from build123d import *

# Parameters (mm, degrees)
SKETCH1_W                  = 35.3
SKETCH1_H                  = 24
BOSS_EXTRUDE1_DEPTH        = 1
F_3_5_3_5_DIAMETER_HOLE1_D = 3.5
SKETCH5_W                  = 7.129651431
SKETCH5_H                  = 6
BOSS_EXTRUDE2_DEPTH        = 0.7


with BuildPart() as part:
    # Sketch1 → Boss-Extrude1 (new body)
    with BuildSketch(Plane(origin=(0, 0, 0), x_dir=(1, 0, 0), z_dir=(0, 1, 0))):
        Rectangle(SKETCH1_W, SKETCH1_H)
    extrude(amount=BOSS_EXTRUDE1_DEPTH)

    # Ø3.5 (3.5) Diameter Hole1 (through all)
    with Locations(Plane(origin=(0, 1, 0), x_dir=(1, 0, 0), z_dir=(0, 1, 0))):
        with Locations((-3.75, 8.7), (14.35, -8.7)):
            Hole(F_3_5_3_5_DIAMETER_HOLE1_D / 2)

    # Sketch5 → Boss-Extrude2 (add)
    with BuildSketch(Plane.XZ):
        with Locations((18.431222248, -1)):
            Rectangle(SKETCH5_W, SKETCH5_H)
    extrude(amount=BOSS_EXTRUDE2_DEPTH)


solid = part.part
For this review, take the finished solid that the model builds, in its own axes (mm). A direction names the side the tool comes from. Give positions to 0.01 mm unless a question says otherwise; leave off trailing zeros. Loops run counter-clockwise (first coordinate to the right, second up) from the corner with the lowest first, then second, coordinate; pieces in that order, holes last. Notation, with made-up numbers: M -38,-28.5 L 7,-28.5 A18 cw 7,-6.5 Z; hole C 75,-11 d3. An arc over 180 degrees is marked long. Put each result on its own line as item: value. Start each with the question number.
(1) Add section C-C, the plane x = 14.35. Write out the cut boundary in (y, z), then the cut area to 3 significant figures.
(2) Add section A-A, the plane z = -8.7. Write out the cut boundary in (x, y).
(3) Add section B-B, the plane y = 0.5. Write out the cut boundary in (x, z), then the cut area to 3 significant figures.
(4) The part is to be moulded in two halves that separate along X. For faces 3 (the cylindrical face through (-2, 0.49, -8.78)), 4 (the flat face through (-17.65, 0.5, 0.2)), 5 (the flat face through (0, 0, 0)), 6 (the cylindrical face through (15.64, 0.49, 7.52)), say which applies: +X half, -X half, draft (parallel to the pull), parting line (faces both ways), or undercut.
(5) Wall thickness on L1, parallel to X at y = 0.85, z = 8.7; L2, parallel to Z at x = 14.35, y = 0.35; L3, parallel to X at y = 0.35, z = 3.5: over which ranges is each line inside the solid? List them lowest first.
(6) For pin 1 (0.6 mm diameter, centred on y = -0.5, z = -1, fed in from -X); pin 2 (4 mm diameter, centred on x = 7, z = -2, fed in from -Y); pin 3 (1.3 mm diameter, centred on x = 19, z = -0.5, fed in from +Y), all flat-tipped, find the tip position at first contact; note any pin that passes through.
(7) Machinability: for faces 1 (the flat face through (-0.2, 0.5, -12)), 2 (the flat face through (20, 0, -1)), which of the approach directions +Z, -Z, +X, -X, +Y, -Y give a long, thin tool a straight path to every point of the face, cutting with its end or side? Answer none if there is none.
(8) Add section D-D, the plane x = 10. Write out the cut boundary in (y, z).
Result:
1. outline: M 0,-12 L 1,-12 L 1,6.95 L 0,6.95 Z; M 0,10.45 L 1,10.45 L 1,12 L 0,12 Z
1. area: 20.5 mm^2
2. outline: M -17.65,0 L -5.5,0 L -5.5,1 L -17.65,1 Z; M -2,0 L 17.65,0 L 17.65,1 L -2,1 Z
3. outline: M -17.65,-12 L 17.65,-12 L 17.65,12 L -17.65,12 Z; hole C -3.75,-8.7 d3.5; hole C 14.35,8.7 d3.5
3. area: 828 mm^2
4. face 3: undercut
4. face 4: -X half
4. face 5: draft
4. face 6: undercut
5. L1: x = -17.65 to 12.6, 16.1 to 17.65
5. L2: z = -12 to 6.95, 10.45 to 12
5. L3: x = -17.65 to 17.65
6. pin 1: stops at x = 14.87
6. pin 2: stops at y = 0
6. pin 3: stops at y = 0
7. face 1: -Z, +X, -X, +Y, -Y
7. face 2: +Z, -Z, +X, +Y
8. outline: M 0,-12 L 1,-12 L 1,12 L 0,12 Z
